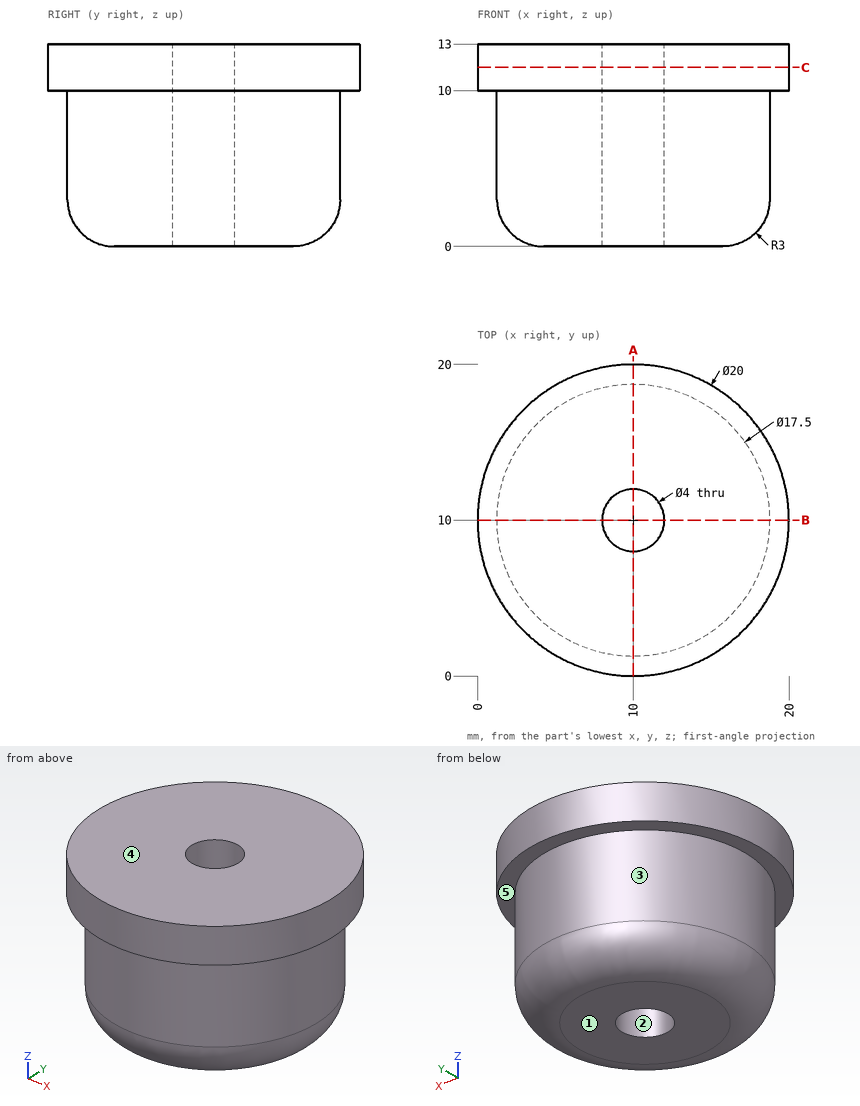
Drawing for the job (mm, zero at the part's lowest x, y, z). A direction names the side the tool comes from. Coordinates: 2 decimals unless noted, no trailing zeros. Order: outer loops, then holes, each group sorted by start corner. A loop starts at its lowest first (then second) coordinate and runs counter-clockwise, first axis right, second up.
Item 1: Pin check, flat tips, straight feed: pin 1 Ø4 at (y, z) = (14.5, 10.5) entering from +X; pin 2 Ø1 at (y, z) = (15.5, 5) entering from +X; pin 3 Ø1.5 at (x, y) = (3, 14) entering from -Z; pin 4 Ø3 at (x, y) = (10, 10) entering from +Z. Stop position of each tip, or through.
Check sheet entries:
pin 1: stops at x = 19.68
pin 2: stops at x = 17.18
pin 3: stops at z = 0.44
pin 4: passes through
Item 2: 3-axis set-ups, long thin cutter, end or side, ignore diameter. For the marked faces 4 and 5: which of +Z, -Z, +X, -X, +Y, -Y reach the whole face in a straight line?
Check sheet entries:
face 4: +Z, +X, -X, +Y, -Y
face 5: -Z
Item 3: Band-saw the part on C-C on z = 11.5. List the corners of the cut face in (x, y).
Check sheet entries:
outline: circle Ø20 at (10, 10); hole circle Ø4 at (10, 10)
Item 4: Drill centre lines: L1, parallel to X at y = 10, z = 3.75; L2, parallel to Z at x = 17.5, y = 16.5. Where is each one in solid material? Low to high.
Check sheet entries:
L1: x = 1.25 to 8, 12 to 18.75
L2: z = 10 to 13
Item 5: Two-plate mould, pull along X, no slides. Class the marked faces 1, 2 and 3: +X half, -X half, draft (parallel to the pull), parting line (faces both ways), or undercut.
Check sheet entries:
face 1: draft
face 2: undercut
face 3: parting line
Item 6: Band-saw the part on A-A on x = 10. List the corners of the cut face in (y, z), plus the area to 3 significant figures.
Check sheet entries:
outline: (0, 10) - (1.25, 10) - (1.25, 3) arc R3 ccw to (4.25, 0) - (8, 0) - (8, 13) - (0, 13) - close; (12, 0) - (15.75, 0) arc R3 ccw to (18.75, 3) - (18.75, 10) - (20, 10) - (20, 13) - (12, 13) - close
area: 179 mm2
